Source: CAD feature listing. Evaluate the final solid. Frame: model axes, mm. A direction names the side the tool comes from. Round coordinates to 2 decimals unless told otherwise and drop trailing zeros. Loops run counter-clockwise (first coordinate to the right, second up) from the corner with the lowest first, then second, coordinate; pieces in that order, holes last. Notation, with made-up numbers: M 51.5,83.25 L 69.5,83.25 A21 ccw 69.5,98.25 Z; hole C -31,-26.5 d10. An arc over 180 degrees is marked long. Write each question's results on one line, items separated by ' | '. Start each with the question number.
1. Ray query, line 1 (Z direction, x = 6.5, y = -281.5); line 2 (Z direction, x = 0, y = -59); line 3 (Y direction, x = 58.5, z = -70). Return the intervals inside material, ascending.
2. Section D-D on y = -141. Output: boundary loops of the cut face in (x, z), and give its area (3 significant figures).
3. Contact query for flat-ended pins moving along their axis: pin 1 Ø1 at (x, y) = (62, -181.5) entering from +Z; pin 2 Ø6 at (x, z) = (-95, -174.5) entering from +Y; pin 3 Ø4 at (y, z) = (-387, -125) entering from -X; pin 4 Ø1 at (y, z) = (-287.5, -17.5) entering from +X. Output: stop coordinate, or through.
4. Section B-B on z = 0. Output: boundary loops of the cut face in (x, y).
5. Set-up query: faces 1 (the flat face through (76, -253, 2)), 2 (the cylindrical face through (60.967, -128.271, -25.278)), 3 (the flat face through (-141, -431, -161)). Return all of +Z, -Z, +X, -X, +Y, -Y with unobstructed straight access to the full face (end or side cutting, diameter ignored); none if empty.
6. Section A-A on x = 0. Output: boundary loops of the cut face in (y, z).
7. Section C-C on x = -167.5. Output: boundary loops of the cut face in (y, z), and give its area (3 significant figures).
8. Draft query along X for faces 4 (the cylindrical face through (126.66, -449.24, -243.53)), 5 (the cylindrical face through (-38.37, -362, -172.79)), 6 (the flat face through (44, 0, 50)). Return one class per face: released by +X, released by -X, zero draft, split by the parting line, or undercut.
from build123d import *

# Parameters (mm, degrees)
F0_R     = 274.5
F1_DEPTH = 468
F2_R     = 66
F3_DEPTH = 468
F4_R     = 177
F4_R_2   = 66
F5_DEPTH = 215
F6_R     = 274.5
F6_R_2   = 213
F7_DEPTH = 431


with BuildPart() as f1:
    # F0 (on Front) → F1 (new body)
    with BuildSketch(Plane.XZ):
        Circle(F0_R)
    extrude(amount=F1_DEPTH)

    # F2 (on face) → F3 (cut)
    with BuildSketch(Plane.XZ.offset(468)):
        Circle(F2_R)
    extrude(amount=-F3_DEPTH, mode=Mode.SUBTRACT)

    # F4 (on face) → F5 (cut)
    with BuildSketch(Plane.XZ.offset(468)):
        Circle(F4_R)
        Circle(F4_R_2, mode=Mode.SUBTRACT)
    extrude(amount=-F5_DEPTH, mode=Mode.SUBTRACT)

    # F6 (on face) → F7 (cut)
    with BuildSketch(Plane(origin=(0, 0, 0), x_dir=(-1, 0, 0), z_dir=(0, 1, 0))):
        Circle(F6_R)
        Circle(F6_R_2, mode=Mode.SUBTRACT)
    extrude(amount=-F7_DEPTH, mode=Mode.SUBTRACT)


solid = f1.part
Taken from the geometry:
1) line 1: -212.9 to -176.88, 176.88 to 212.9 | line 2: -213 to -66, 66 to 213 | line 3: -253 to 0
2) outline: C 0,0 d426; hole C 0,0 d132 | area: 129,000 mm^2
3) pin 1: z = 203.93 | pin 2: y = 0 | pin 3: x = -173.9 | pin 4: x = 212.32
4) outline: M -274.5,-468 L -177,-468 L -177,-253 L -66,-253 L -66,0 L -213,0 L -213,-431 L -274.5,-431 Z; M 66,-253 L 177,-253 L 177,-468 L 274.5,-468 L 274.5,-431 L 213,-431 L 213,0 L 66,0 Z
5) face 1: -Y | face 2: +Y, -Y | face 3: +Y
6) outline: M -468,-274.5 L -431,-274.5 L -431,-213 L 0,-213 L 0,-66 L -253,-66 L -253,-177 L -468,-177 Z; M -468,177 L -253,177 L -253,66 L 0,66 L 0,213 L -431,213 L -431,274.5 L -468,274.5 Z
7) outline: M -468,-217.47 L -431,-217.47 L -431,-131.58 L 0,-131.58 L 0,131.58 L -431,131.58 L -431,217.47 L -468,217.47 L -468,57.21 L -253,57.21 L -253,-57.21 L -468,-57.21 Z | area: 105,000 mm^2
8) face 4: split by the parting line | face 5: undercut | face 6: zero draft
